The drawing under review shows one solid part. Ordinate dimensions are in mm from its lowest x, y, z. Give positions to 0.01 mm unless a question says otherwise; leave off trailing zeros. Write each loop counter-clockwise with the first axis right and the second up, starting at its lowest first coordinate (ties: lowest second). Pieces come first, ordered by that corner, then holes. Notation, with made-up numbers: (-8.75, 34.5) -> (37.25, 34.5) arc R19 ccw to (37.25, 61.5) -> close; hole circle Ø8 at (56.25, 3). An arc over 180 degrees is marked (long way). Use CSV: the item, a comma, the result in double quotes.
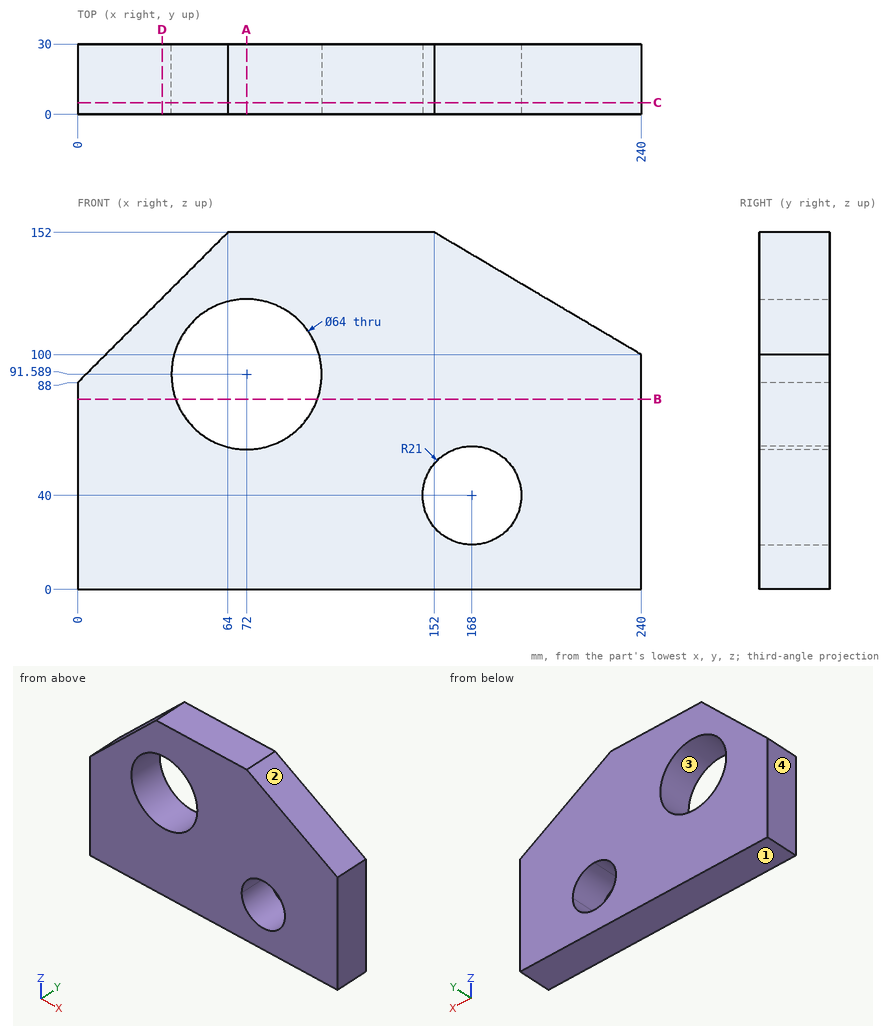
(1) Take a section at D-D (x = 36). Write out the cut boundary in (y, z), then the cut area to 3 significant figures.
Established:
outline,"(0, 0) -> (30, 0) -> (30, 124) -> (0, 124) -> close"
area,"3,720 mm2"
(2) Take a section at B-B (z = 81). Write out the cut boundary in (x, y).
Established:
outline,"(0, 0) -> (41.8, 0) -> (41.8, 30) -> (0, 30) -> close; (102.2, 0) -> (240, 0) -> (240, 30) -> (102.2, 30) -> close"
(3) Take a section at A-A (x = 72). Write out the cut boundary in (y, z).
Established:
outline,"(0, 0) -> (30, 0) -> (30, 59.59) -> (0, 59.59) -> close; (0, 123.59) -> (30, 123.59) -> (30, 152) -> (0, 152) -> close"
(4) Clearance check with a flat-ended pin moving along its axis: pin 1 (12 mm diameter, centred on x = 178, y = 11, fed in from +Z). State where the tip first meets the part, or that it passes through.
Established:
pin 1,"stops at z = 140.18"
(5) Mouldability with a two-part tool opening along Z and no side actions: class the marked faces 1, 2, 3 and 4 as +Z half, -Z half, draft (parallel to the pull), parting line (faces both ways), or undercut.
Established:
face 1,"-Z half"
face 2,"+Z half"
face 3,"undercut"
face 4,"draft"
(6) For line 1 along Z through (x, y) = (72, 13); line 2 along X through (y, z) = (4.75, 22) (1 decimal); line 3 along X through (y, z) = (20.5, 95), list the stretches that pass through material, from the lowest coordinate up. Write a range as [from, to].
Established:
line 1,"z = [0, 59.59], [123.59, 152]"
line 2,"x = [0, 157.2], [178.8, 240]"
line 3,"x = [7, 40.18], [103.82, 240]"
(7) Take a section at C-C (y = 5). Write out the cut boundary in (x, z), then the cut area to 3 significant figures.
Established:
outline,"(0, 0) -> (240, 0) -> (240, 100) -> (152, 152) -> (64, 152) -> (0, 88) -> close; hole circle Ø64 at (72, 91.59); hole (147, 40) arc R21 ccw to (189, 40) arc R21 ccw to (168, 61) arc R21 ccw to start"
area,"27,500 mm2"
